Read the model definition and answer for the solid it produces. Units are mm, in the model's axes. A direction names the side the tool comes from. Coordinates: 2 decimals unless noted, no trailing zeros. Write each loop counter-clockwise with the first axis right and the second up, starting at its lowest first coordinate (ties: lowest second). Pieces come first, ordered by that corner, then holes.
(1) The part is cut by section C-C, the plane x = -1.5. Determine the outline of the cut face in (y, z), and give its area (3 significant figures).
(2) Straight lines are drawn through the part: line 1 along Y through (x, z) = (0, 14.65); line 2 along Z through (x, y) = (13, 6); line 3 along X through (y, z) = (1.5, 9). For each, find the intervals that lie inside material, in ascending order.
(3) Which of the six approach directions +Z, -Z, +X, -X, +Y, -Y give full straight-line access (tool end or side, diameter ignored) to faces 4 (the flat face through (15, 15, 23.5)), 5 (the flat face through (7.5, -17, 13)), 6 (the flat face through (15, 15, 19.5)), 7 (the flat face through (15.935, 20.177, 1.972))?
(4) Given pin 1 (4 mm diameter, centred on y = -15, z = 14, fed in from -X); pin 2 (10.5 mm diameter, centred on x = 19.5, y = 18.5, fed in from +Z); pin 3 (7.5 mm diameter, centred on x = 0.5, y = -25.5, fed in from -Z), each flat-ended and moving along its own axis, determine where each tip first touches the part or whether it passes through.
(5) The part is cut by section A-A, the plane y = 15. Determine the outline of the cut face in (x, z), and give its area (3 significant figures).
(6) The part is cut by section B-B, the plane z = 2. Determine the outline of the cut face in (x, y).
(7) The part is cut by section D-D, the plane z = 7.75. Determine the outline of the cut face in (x, y), and give its area (3 significant figures).
(8) Determine the mould class of faces 1 (the flat face through (12, 15, 4)), 2 (the cylindrical face through (21.97, 21.87, 1.97)), 3 (the flat face through (9.896, 17.674, 21.472)) for opening direction Y: pulls with the +Y half, pulls with the -Y half, needs draft (parallel to the pull), parting line crosses it, or undercut.
```python
from build123d import *

# Parameters (mm, degrees)
EXTRUDE_1_DEPTH     = 25
SKETCH_1_4_R        = 3
EXTRUDE_3_DEPTH     = 4
EXTRUDE_START       = -4
EXTRUDE_4_DEPTH     = 4
SKETCH_3_R          = 3
CUT_EXTRUDE_1_DEPTH = 41.747119864
CUT_EXTRUDE_2_REACH = 45.647
SKETCH_5_R          = 7.5
SKETCH_5_R_2        = 4
EXTRUDE_5_DEPTH     = 3.5


with BuildPart() as part:
    # Sketch 1 → Extrude 1 (new body)
    with BuildSketch(Plane.XY):
        with BuildLine():
            ThreePointArc((7.494638572, -0.283536021), (-5.303300859, -5.303300859), (-0.283536021, 7.494638572))
            Line((-0.283536021, 7.494638572), (4.048166637, 11.82634123))
            ThreePointArc((4.048166637, 11.82634123), (-10.169859462, -7.268009254), (12.5, 0))
            ThreePointArc((12.5, 0), (12.330435219, 2.05191796), (11.82634123, 4.048166637))
            Line((11.82634123, 4.048166637), (7.494638572, -0.283536021))
        make_face()
        with BuildLine():
            Line((4.048166637, 11.82634123), (-0.283536021, 7.494638572))
            ThreePointArc((-0.283536021, 7.494638572), (5.202089957, 5.40261604), (7.5, 0))
            ThreePointArc((7.5, 0), (7.498659523, -0.141793353), (7.494638572, -0.283536021))
            Line((7.494638572, -0.283536021), (11.82634123, 4.048166637))
            ThreePointArc((11.82634123, 4.048166637), (8.838834765, 8.838834765), (4.048166637, 11.82634123))
        make_face()
    extrude(amount=EXTRUDE_1_DEPTH)

    # Sketch 1_4 → Extrude 3 (add)
    with BuildSketch(Plane.XY):
        with BuildLine():
            Line((15.909902577, 23.68807717), (4.048166637, 11.82634123))
            ThreePointArc((4.048166637, 11.82634123), (8.838834765, 8.838834765), (11.82634123, 4.048166637))
            Line((11.82634123, 4.048166637), (23.68807717, 15.909902577))
            ThreePointArc((23.68807717, 15.909902577), (23.68807717, 23.68807717), (15.909902577, 23.68807717))
        make_face()
        with Locations((19.798989873, 19.798989873)):
            Circle(SKETCH_1_4_R, mode=Mode.SUBTRACT)
    extrude(amount=EXTRUDE_3_DEPTH)

    # Sketch 2 → Extrude 4 (add)
    with BuildSketch(Plane.XY.offset(23.5).offset(EXTRUDE_START)):
        with BuildLine():
            Line((4.048166637, 11.82634123), (15.909902577, 23.68807717))
            ThreePointArc((15.909902577, 23.68807717), (23.68807717, 23.68807717), (23.68807717, 15.909902577))
            Line((23.68807717, 15.909902577), (11.82634123, 4.048166637))
            ThreePointArc((11.82634123, 4.048166637), (8.838834765, 8.838834765), (4.048166637, 11.82634123))
        make_face()
    extrude(amount=EXTRUDE_4_DEPTH)

    # Sketch 3 → Cut-Extrude 1 (cut, through all)
    with BuildSketch(Plane(origin=(0, 0, 19.5), x_dir=(-1, 0, 0), z_dir=(0, 0, -1))):
        with Locations(Location((-19.798989873, 19.798989873, 0), (0, 0, 180))):
            Circle(SKETCH_3_R)
    extrude(amount=-CUT_EXTRUDE_1_DEPTH, mode=Mode.SUBTRACT)

    # Sketch 4 → Cut-Extrude 2 (cut, up to next)
    with BuildSketch(Plane(origin=(0, 0, 0), x_dir=(-1, 0, 0), z_dir=(0, 0, -1)), mode=Mode.PRIVATE) as cut_extrude_2_sk1:
        with BuildLine():
            Line((-17.67766953, 21.920310217), (-14.142135624, 18.384776311))
            ThreePointArc((-14.142135624, 18.384776311), (-14.142135624, 14.142135624), (-18.384776311, 14.142135624))
            Line((-18.384776311, 14.142135624), (-21.920310217, 17.67766953))
            ThreePointArc((-21.920310217, 17.67766953), (-21.920310217, 21.920310217), (-17.67766953, 21.920310217))
        make_face()
    cut_extrude_2_tool1 = extrude(cut_extrude_2_sk1.sketch, amount=-CUT_EXTRUDE_2_REACH, mode=Mode.PRIVATE) & part.part
    add(cut_extrude_2_tool1.solids().sort_by_distance((18.031223, 18.031223, 0))[0], mode=Mode.SUBTRACT)

    # Sketch 5 → Extrude 5 (add, symmetric)
    # profile 1 of 2: a face of its own
    with BuildSketch(Plane.XY.offset(12.5)):
        with Locations((0, -23)):
            Circle(SKETCH_5_R)
        with Locations((0, -23)):
            Circle(SKETCH_5_R_2, mode=Mode.SUBTRACT)
    # profile 2 of 2: a face of its own
    with BuildSketch(Plane.XY.offset(12.5)):
        with BuildLine():
            ThreePointArc((-7.5, -23), (0, -15.5), (7.5, -23))
            Line((7.5, -23), (7.5, -10))
            Line((7.5, -10), (-7.5, -10))
            Line((-7.5, -10), (-7.5, -23))
        make_face()
    extrude(amount=EXTRUDE_5_DEPTH, both=True)


solid = part.part
```
Computed:
1. outline: (-30.35, 9) - (-26.71, 9) - (-26.71, 16) - (-30.35, 16) - close; (-19.29, 9) - (-12.41, 9) - (-12.41, 0) - (-7.35, 0) - (-7.35, 25) - (-12.41, 25) - (-12.41, 16) - (-19.29, 16) - close; (7.35, 0) - (12.41, 0) - (12.41, 25) - (7.35, 25) - close
1. area: 327 mm2
2. line 1: y = -30.5 to -27, -19 to -7.5, 7.5 to 12.5
2. line 2: z = 0 to 4, 19.5 to 23.5
2. line 3: x = -12.41 to -7.35, 7.35 to 12.41
3. face 4: +Z, +X, +Y
3. face 5: +Z, -Z, +X, -Y
3. face 6: +X, +Y
3. face 7: -Z
4. pin 1: stops at x = -7.5
4. pin 2: stops at z = 23.5
4. pin 3: stops at z = 9
5. outline: (7.22, 0) - (13.54, 0) - (13.54, 4) - (7.22, 4) - close; (7.22, 19.5) - (22.78, 19.5) - (22.78, 23.5) - (7.22, 23.5) - close; (19.24, 0) - (22.78, 0) - (22.78, 4) - (19.24, 4) - close
5. area: 102 mm2
6. outline: (4.05, 11.83) arc R12.5 ccw (long way) to (11.83, 4.05) - (23.69, 15.91) arc R5.5 ccw to (15.91, 23.69) - close; hole (7.49, -0.28) arc R7.5 ccw to (7.5, 0) arc R7.5 ccw (long way) to start; hole (14.14, 18.38) arc R3 ccw to (18.38, 14.14) - (21.92, 17.68) arc R3 ccw to (17.68, 21.92) - close
7. outline: circle Ø25 at (0, 0); hole (7.49, -0.28) arc R7.5 ccw to (7.5, 0) arc R7.5 ccw (long way) to start
7. area: 314 mm2
8. face 1: needs draft
8. face 2: undercut
8. face 3: pulls with the +Y half
